Could you check a few things on this drawing? It's one solid part, dimensions in mm from its lowest x, y, z. Give positions to 0.01 mm unless a question says otherwise; leave off trailing zeros. Loops run counter-clockwise (first coordinate to the right, second up) from the corner with the lowest first, then second, coordinate; pieces in that order, holes last. Notation, with made-up numbers: M -29,-9.75 L 24,-9.75 A5 cw 24,-0.75 Z; hole C 87.25,78 d1. An arc over 180 degrees is marked long. Answer as a JSON object with one key per item and string values.
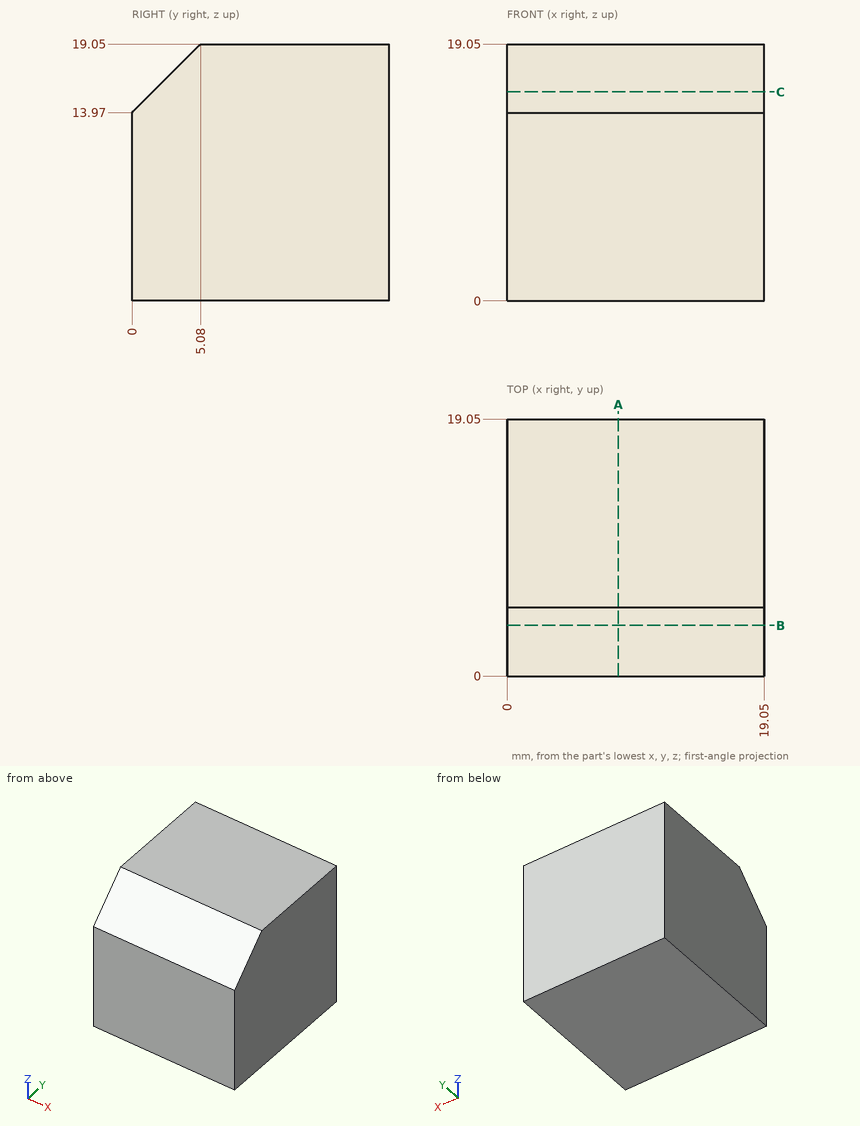
1) Suppose I cut it at C-C, the plane z = 15.5. Write out the boundary of the cut face in (x, y), and give its area (3 significant figures).
Answer list:
{"outline": "M 0,1.53 L 19.05,1.53 L 19.05,19.05 L 0,19.05 Z", "area": "334 mm^2"}
2) Please list where these lines run through material, in increasing order: line 1 along Y through (x, z) = (14.25, 15.75); line 2 along Y through (x, z) = (13.75, 16.25); line 3 along Z through (x, y) = (4.75, 2). Write a range as from..to.
Answer list:
{"line 1": "1.78..19.05", "line 2": "2.28..19.05", "line 3": "0..15.97"}
3) Suppose I cut it at B-B, the plane y = 3.75. Write out the boundary of the cut face in (x, z), and give its area (3 significant figures).
Answer list:
{"outline": "M 0,0 L 19.05,0 L 19.05,17.72 L 0,17.72 Z", "area": "338 mm^2"}
4) Suppose I cut it at A-A, the plane x = 8.25. Write out the boundary of the cut face in (y, z).
Answer list:
{"outline": "M 0,0 L 19.05,0 L 19.05,19.05 L 5.08,19.05 L 0,13.97 Z"}
